Solid Edge part; units mm, degrees
sketch "Sketch1" plane through (0, 0, 0) normal (0, 0, 1) x (1, 0, 0)
  arc A0 (0, 16) -> (1, 15) centre (1, 16) ccw
  line L0 (1, 15) -> (12, 15)
  arc A1 (12, 15) -> (13, 16) centre (12, 16) ccw
  line L1 (13, 16) -> (13, 18.667)
  arc A2 (13, 18.667) -> (12.667, 19) centre (12.667, 18.667) ccw
  line L2 (12.667, 19) -> (9.2743, 19)
  arc A3 (9.2743, 19) -> (3.7257, 19) centre (6.5, 21.25) cw
  line L3 (3.7257, 19) -> (0.333, 19)
  arc A4 (0.333, 19) -> (0, 18.667) centre (0.333, 18.667) ccw
  line L4 (0, 18.667) -> (0, 16)
revolve "RevolvedProtrusion1" add sketch "Sketch1" angle 360 about axis through (12, 0, 0) along (-1, 0, 0)
properties material "Steel"
Here's how the part is built. I have some questions about the finished solid (model axes, mm). Coordinates: 2 decimals unless noted, no trailing zeros. Loops run counter-clockwise (first coordinate to the right, second up) from the corner with the lowest first, then second, coordinate; pieces in that order, holes last. Notation, with made-up numbers: (-32, 46) - (-13, 46) arc R25 cw to (-13, 71) - close; hole circle Ø3 at (-12, -22.5). An arc over 180 degrees is marked (long way). Answer as CSV lines item,"result".
Q1. We'd pull the mould along Y, two halves only. Please class faces 1 (the face through (0, 15, -6)), 2 (the face through (6.577, -14.985, 0.66)), 3 (the face through (10.947, 8.767, 16.856)): pulls with the +Y half, pulls with the -Y half, needs draft (parallel to the pull), parting line crosses it, or undercut.
Response:
face 1,"needs draft"
face 2,"undercut"
face 3,"parting line crosses it"
Q2. For pin 1 (4 mm diameter, centred on x = 9.5, y = 3, fed in from -Z); pin 2 (5 mm diameter, centred on x = 2, z = 1, fed in from +Y); pin 3 (5 mm diameter, centred on x = 4.5, z = 14.5, fed in from -Y), each with a flat end and sliding along its axis, tell me the tip position at first contact or that it passes through.
Response:
pin 1,"z = -18.97"
pin 2,"y = 19"
pin 3,"y = -14.63"
Q3. If we section it at C-C, the plane x = 3: Write out the boundary of the cut face in (y, z).
Response:
outline,"circle Ø38 at (0, 0); hole circle Ø30 at (0, 0)"
Q4. If I drill on L1, parallel to Y at x = 9.75, z = 0; L2, parallel to Y at x = 6.5, z = -1, over which ranges is the centre line in solid material (lowest first)? Write a range as [from, to].
Response:
L1,"[-19, -15], [15, 19]"
L2,"[-17.65, -14.97], [14.97, 17.65]"
Q5. If we section it at A-A, the plane y = 0: Write out the boundary of the cut face in (x, z), and give its area (3 significant figures).
Response:
outline,"(0, -18.67) arc R0.33 ccw to (0.33, -19) - (3.73, -19) arc R3.57 cw to (9.27, -19) - (12.67, -19) arc R0.33 ccw to (13, -18.67) - (13, -16) arc R1 ccw to (12, -15) - (1, -15) arc R1 ccw to (0, -16) - close; (0, 16) arc R1 ccw to (1, 15) - (12, 15) arc R1 ccw to (13, 16) - (13, 18.67) arc R0.33 ccw to (12.67, 19) - (9.27, 19) arc R3.57 cw to (3.73, 19) - (0.33, 19) arc R0.33 ccw to (0, 18.67) - close"
area,"92.8 mm2"
Q6. If we section it at D-D, the plane x = 5.25: Write out the boundary of the cut face in (y, z).
Response:
outline,"circle Ø35.81 at (0, 0); hole circle Ø30 at (0, 0)"
